from build123d import *

# Parameters (mm, degrees)
SKETCH_1_W                  = 43
SKETCH_1_H                  = 47
EXTRUDE_1_DEPTH             = 1
SKETCH_2_W                  = 43
SKETCH_2_H                  = 122
EXTRUDE_2_DEPTH             = 3
SKETCH_3_W                  = 43
SKETCH_3_H                  = 122
EXTRUDE_3_DEPTH             = 3
SKETCH_5_R                  = 2.25
CUT_EXTRUDE_1_DEPTH         = 10
PATTERN_LINEAR_1_COUNT      = 2
PATTERN_LINEAR_1_PITCH      = 34
PATTERN_LINEAR_1_COUNT_DIR2 = 2
PATTERN_LINEAR_1_PITCH_DIR2 = 34
SKETCH_6_W                  = 43
SKETCH_6_H                  = 53
EXTRUDE_4_DEPTH             = 3.5
HOLE_WIZARD_M3_1_D          = 2.5
HOLE_WIZARD_M3_1_DEPTH      = 7.5
HOLE_WIZARD_M3_1_TIP        = 0.751075774


with BuildPart() as part:
    # 草图1 → 凸台-拉伸1 (new body)
    with BuildSketch(Plane.XY):
        Rectangle(SKETCH_1_W, SKETCH_1_H)
    extrude(amount=EXTRUDE_1_DEPTH)

    # 草图2 → 凸台-拉伸2 (add)
    with BuildSketch(Plane(origin=(0, 23.5, 0), x_dir=(1, 0, 0), z_dir=(0, 1, 0))):
        with Locations((0, 60)):
            Rectangle(SKETCH_2_W, SKETCH_2_H)
    extrude(amount=EXTRUDE_2_DEPTH)

    # 草图3 → 凸台-拉伸3 (add)
    with BuildSketch(Plane.XZ.offset(23.5)):
        with Locations((0, -60)):
            Rectangle(SKETCH_3_W, SKETCH_3_H)
    extrude(amount=EXTRUDE_3_DEPTH)

    # 草图5 → 切除-拉伸1 (cut)
    with BuildSketch(Plane.XY.offset(1)):
        with Locations((-17, -17)):
            Circle(SKETCH_5_R)
    cut_extrude_1 = extrude(amount=-CUT_EXTRUDE_1_DEPTH, mode=Mode.SUBTRACT)

    # 阵列(线性)1: Cut-Extrude 1 2 × 2
    with Locations(*[(j * PATTERN_LINEAR_1_PITCH_DIR2, i * PATTERN_LINEAR_1_PITCH, 0) for i in range(PATTERN_LINEAR_1_COUNT) for j in range(PATTERN_LINEAR_1_COUNT_DIR2) if (i, j) != (0, 0)]):
        add(cut_extrude_1, mode=Mode.SUBTRACT)

    # 草图6 → 凸台-拉伸4 (add)
    with BuildSketch(Plane(origin=(0, 0, -121), x_dir=(-1, 0, 0), z_dir=(0, 0, -1))):
        Rectangle(SKETCH_6_W, SKETCH_6_H)
    extrude(amount=EXTRUDE_4_DEPTH)

    # M3 螺纹孔1
    with Locations(Plane(origin=(-15.5, 17.5, -121), x_dir=(1, 0, 0), z_dir=(0, 0, 1))):
        with Locations((0, 0), (31, 0), (0, -35), (31, -35)):
            Hole(HOLE_WIZARD_M3_1_D / 2, depth=HOLE_WIZARD_M3_1_DEPTH)
            with Locations((0, 0, -(HOLE_WIZARD_M3_1_DEPTH + HOLE_WIZARD_M3_1_TIP / 2))):  # 118° drill point
                Cone(0, HOLE_WIZARD_M3_1_D / 2, HOLE_WIZARD_M3_1_TIP, mode=Mode.SUBTRACT)


solid = part.part
Could you check a few things on this model? Use its own coordinates, in mm. A direction names the side the tool comes from. Give positions to 0.01 mm unless a question says otherwise; leave off trailing zeros. Write each loop counter-clockwise with the first axis right and the second up, starting at its lowest first coordinate (ties: lowest second). Pieces come first, ordered by that corner, then holes. Notation, with made-up numbers: (-27, 0) -> (-4, 0) arc R10 ccw to (-4, 14) -> close; hole circle Ø8 at (37.25, -15). An arc over 180 degrees is marked (long way). Write each question's results on one line, items separated by ' | '. Start each with the question number.
Q1. I'm going to push flat-ended pins straight in: pin 1 Ø4 at (x, y) = (17, -17) entering from +Z; pin 2 Ø1.5 at (x, y) = (-15.5, -17.5) entering from -Z. Where does each tip first touch, or does it pass through?
Q2. I need wall thicknesses on probe 1 along Y at (x, z) = (-17, 0.55); probe 2 along Y at (x, z) = (15.5, -122.55); probe 3 along Z at (x, y) = (10, 15.5). Which ranges of each line are inside material? Lowest first, please.
Q3. Suppose I cut it at A-A, the plane y = -21.5. List the corners of the cut face in (x, z) for me, and give its area (4 significant figures).
Q4. We'd pull the mould along X, two halves only. Please class faces 1 (the face through (-21.5, -24, -75)), 2 (the face through (0, 0, -121)), 3 (the face through (18.038, 15.004, 0.507)): +X half, -X half, draft (parallel to the pull), parting line (faces both ways), or undercut.
Q5. Suppose I cut it at B-B, the plane z = -108.5. List the corners of the cut face in (x, y) for me, and give its area (3 significant figures).
Q6. Which directions (+Z, -Z, +X, -X, +Y, -Y) give clear straight access to the entire face, cutting with the end or side of a thin tool? Please do faces 4 (the face through (-14.579, -16.655, -122.774)), 5 (the face through (0, 0, 0)), 6 (the face through (-15.962, 15.004, 0.507)), 7 (the face through (0, -26.5, -61)).
Q7. Suppose I cut it at C-C, the plane x = -7. List the corners of the cut face in (y, z) for me.
Outcome:
1) pin 1: z = -121 | pin 2: z = 0
2) probe 1: -26.5 to -19.25, -14.75 to 14.75, 19.25 to 26.5 | probe 2: -26.5 to -18.75, -16.25 to 16.25, 18.75 to 26.5 | probe 3: -124.5 to -121, 0 to 1
3) outline: (-21.5, -124.5) -> (21.5, -124.5) -> (21.5, -121) -> (-21.5, -121) -> close; (-21.5, 0) -> (21.5, 0) -> (21.5, 1) -> (-21.5, 1) -> close | area: 193.5 mm2
4) face 1: -X half | face 2: draft | face 3: undercut
5) outline: (-21.5, -26.5) -> (21.5, -26.5) -> (21.5, -23.5) -> (-21.5, -23.5) -> close; (-21.5, 23.5) -> (21.5, 23.5) -> (21.5, 26.5) -> (-21.5, 26.5) -> close | area: 258 mm2
6) face 4: -Z | face 5: +X, -X | face 6: +Z | face 7: +Z, -Z, +X, -X, -Y
7) outline: (-26.5, -124.5) -> (26.5, -124.5) -> (26.5, 1) -> (-26.5, 1) -> close; hole (-23.5, -121) -> (23.5, -121) -> (23.5, 0) -> (-23.5, 0) -> close
